For this review, take the finished solid that the model builds, in its own axes (mm). Face numbers are marked on the shaded views. A direction names the side the tool comes from. Coordinates: 2 decimals unless noted, no trailing zeros. Write each loop counter-clockwise with the first axis right and the second up, starting at its lowest first coordinate (ties: lowest second). Pieces come first, ordered by that corner, then holes.
1) We need section D-D on x = 23. Write out the cut boundary in (y, z).
2) We need section B-B on z = 4. Write out the cut boundary in (x, y).
3) We need section C-C on y = 5. Write out the cut boundary in (x, z), then the cut area to 3 significant figures.
4) For the marked faces 1, 2 and 3, list the 3-axis set-ups (+Z, -Z, +X, -X, +Y, -Y) from which the entire face can be reached by the end or side of a thin tool; tool diameter is ignored.
5) To check wall thickness, follow line 1 along Y through (x, z) = (0, 24); line 2 along Z through (x, y) = (10.5, 8.5); line 3 along Y through (x, z) = (0, 26.5). State the ranges of each line that lie inside material, in increasing order.
6) We need section A-A on x = 0. Write out the cut boundary in (y, z), then the cut area to 3 significant figures.
7) Insertion check: P1, Ø3, axis at x = -22.5, y = -1.5, coming from the +Z side; P2, Ø1.5, axis at y = 5, z = 14, coming from the +X side; P3, Ø0.9, axis at y = 4.5, z = -30, coming from the -X side; P4, Ø8, axis at x = -18, z = 9, coming from the -Y side. Each pin has a flat end and moves straight along its axis. Give the tip position at first contact, or say it passes through.
8) Mouldability with a two-part tool opening along Z and no side actions: class the marked faces 4, 5, 6 and 7 as pulls with the +Z half, pulls with the -Z half, needs draft (parallel to the pull), parting line crosses it, or undercut.
from build123d import *

# Parameters (mm, degrees)
BOSS_EXTRUDE1_DEPTH            = 20
CUT_EXTRUDE1_DEPTH             = 27.5
CBORE_FOR_M3_SHCS1_D           = 3.4
CBORE_FOR_M3_SHCS1_DEPTH       = 5
CBORE_FOR_M3_SHCS1_CBORE_D     = 6.5
CBORE_FOR_M3_SHCS1_CBORE_DEPTH = 3
FILLET1_R                      = 2


with BuildPart() as part:
    # Sketch1 → Boss-Extrude1 (new body, symmetric)
    with BuildSketch(Plane(origin=(0, 0, 0), x_dir=(1, 0, 0), z_dir=(0, 1, 0))):
        with BuildLine():
            Line((-15, -28.348661632), (15, -28.348661632))
            ThreePointArc((15, -28.348661632), (34.752533521, 3), (15, 34.348661632))
            Line((15, 34.348661632), (-15, 34.348661632))
            ThreePointArc((-15, 34.348661632), (-34.752533521, 3), (-15, -28.348661632))
        make_face()
        with BuildLine():
            Line((-10, -23.348661632), (10, -23.348661632))
            ThreePointArc((10, -23.348661632), (0, 25.4), (-10, -23.348661632))
        make_face(mode=Mode.SUBTRACT)
    extrude(amount=BOSS_EXTRUDE1_DEPTH, both=True)

    # Sketch3 → Cut-Extrude1 (cut)
    with BuildSketch(Plane(origin=(0, 20, 0), x_dir=(1, 0, 0), z_dir=(0, 1, 0))):
        Polygon((-10, 34.348661632), (-10, 31.348661632), (-12.5, 31.348661632), (-12.5, 28.348661632), (12.5, 28.348661632), (12.5, 31.348661632), (10, 31.348661632), (10, 34.348661632), align=None)
    extrude(amount=-CUT_EXTRUDE1_DEPTH, mode=Mode.SUBTRACT)

    # CBORE for M3 SHCS1
    with Locations(Plane.XY.offset(28.348661632)):
        with Locations((0, 10), (0, -10)):
            CounterBoreHole(CBORE_FOR_M3_SHCS1_D / 2, CBORE_FOR_M3_SHCS1_CBORE_D / 2, CBORE_FOR_M3_SHCS1_CBORE_DEPTH, depth=CBORE_FOR_M3_SHCS1_DEPTH)

    # Fillet1
    fillet1_edges = [part.edges().sort_by_distance(p)[0] for p in [
        (10, -7.5, -32.848661632),
        (12.5, -7.5, -29.848661632),
        (-12.5, -7.5, -29.848661632),
        (-10, -7.5, -32.848661632),
    ]]
    fillet(fillet1_edges, radius=FILLET1_R)


solid = part.part
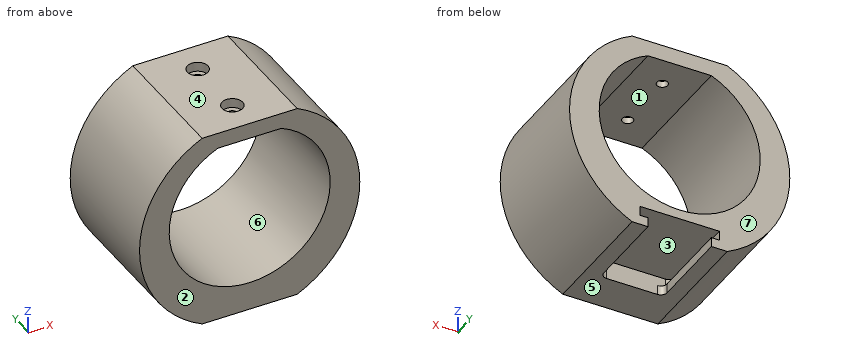
Result:
1. outline: (-20, -29.05) - (20, -29.05) - (20, -10.78) - (-20, -10.78) - close; (-20, 10.78) - (20, 10.78) - (20, 23.05) - (-20, 23.05) - close
2. outline: (-34.04, -20) - (-25.08, -20) - (-25.08, 20) - (-34.04, 20) - close; (25.08, -20) - (34.04, -20) - (34.04, 20) - (25.08, 20) - close
3. outline: (-15, -34.35) - (-10, -34.35) - (-10, -31.35) - (-12.5, -31.35) - (-12.5, -28.35) - (12.5, -28.35) - (12.5, -31.35) - (10, -31.35) - (10, -34.35) - (15, -34.35) arc R34.75 ccw to (15, 28.35) - (-15, 28.35) arc R34.75 ccw to start; hole (-10, 23.35) arc R25.4 ccw (long way) to (10, 23.35) - close
3. area: 1,520 mm2
4. face 1: +Y, -Y
4. face 2: +Z, -Z, +X, -X, -Y
4. face 3: +Y
5. line 1: y = -20 to -11.7, -8.3 to 8.3, 11.7 to 20
5. line 2: z = -34.35 to -31.35, -28.35 to -23.13, 23.13 to 28.35
5. line 3: y = -20 to -13.25, -6.75 to 6.75, 13.25 to 20
6. outline: (-20, -34.35) - (-7.5, -34.35) - (-7.5, -28.35) - (20, -28.35) - (20, -25.4) - (-20, -25.4) - close; (-20, 23.35) - (-11.7, 23.35) - (-11.7, 25.35) - (-13.25, 25.35) - (-13.25, 28.35) - (-20, 28.35) - close; (-8.3, 23.35) - (8.3, 23.35) - (8.3, 25.35) - (6.75, 25.35) - (6.75, 28.35) - (-6.75, 28.35) - (-6.75, 25.35) - (-8.3, 25.35) - close; (11.7, 23.35) - (20, 23.35) - (20, 28.35) - (13.25, 28.35) - (13.25, 25.35) - (11.7, 25.35) - close
6. area: 340 mm2
7. P1: stops at z = 24.69
7. P2: stops at x = 30.72
7. P3: stops at x = -22.42
7. P4: passes through
8. face 4: pulls with the +Z half
8. face 5: pulls with the -Z half
8. face 6: undercut
8. face 7: needs draft
